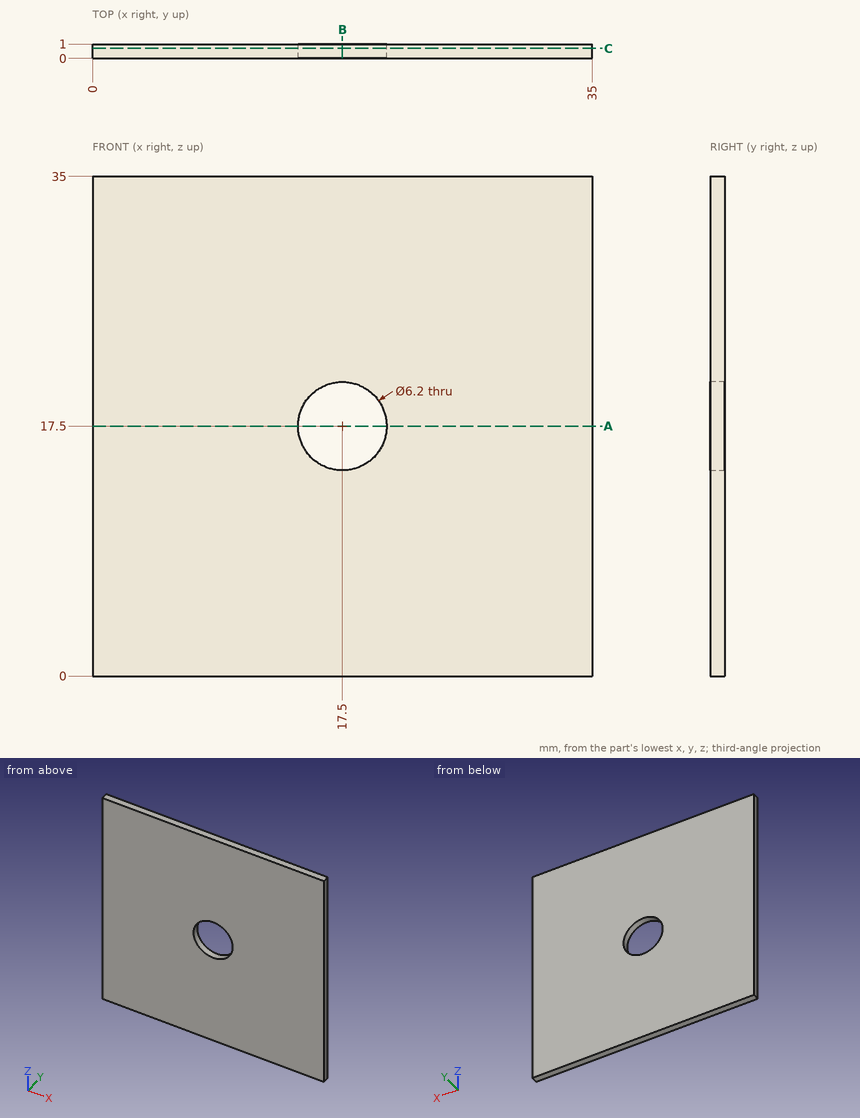
Print and shaded views of the part. All mm, measured from the part's lowest x, y and z. Give positions to 0.01 mm unless a question says otherwise; leave off trailing zeros. Write each loop counter-clockwise with the first axis right and the second up, starting at its lowest first coordinate (ties: lowest second). Pieces come first, ordered by that corner, then holes. Notation, with made-up numbers: (88, -14.5) -> (147, -14.5) arc R9 cw to (147, -10.5) -> close; hole circle Ø4 at (22.5, -39). An arc over 180 degrees is marked (long way). Write item = value, one per line.
(1) Slice it at C-C, the plane y = 0.7. Give the cut face in (x, z), then the cut area to 3 significant figures.
Determined:
outline = (0, 0) -> (35, 0) -> (35, 35) -> (0, 35) -> close; hole circle Ø6.2 at (17.5, 17.5)
area = 1,190 mm2
(2) Probe line 1 along X through (y, z) = (0.5, 17.5); line 2 along Z through (x, y) = (18, 0.3); line 3 along Z through (x, y) = (19, 0.6). List the from-to ranges inside material, lowest first.
Determined:
line_1 = 0 to 14.4, 20.6 to 35
line_2 = 0 to 14.44, 20.56 to 35
line_3 = 0 to 14.79, 20.21 to 35
(3) Slice it at B-B, the plane x = 17.5. Give the cut face in (y, z), then the cut area to 3 significant figures.
Determined:
outline = (0, 0) -> (1, 0) -> (1, 14.4) -> (0, 14.4) -> close; (0, 20.6) -> (1, 20.6) -> (1, 35) -> (0, 35) -> close
area = 28.8 mm2
(4) Slice it at A-A, the plane z = 17.5. Give the cut face in (x, y).
Determined:
outline = (0, 0) -> (14.4, 0) -> (14.4, 1) -> (0, 1) -> close; (20.6, 0) -> (35, 0) -> (35, 1) -> (20.6, 1) -> close
